Read the model definition and answer for the solid it produces. Units are mm, in the model's axes. Coordinates: 2 decimals unless noted, no trailing zeros. Write each loop counter-clockwise with the first axis right and the second up, starting at its lowest first coordinate (ties: lowest second). Pieces come first, ordered by that corner, then holes.
(1) The mould has two halves that part along X. Classify faces 1 (the flat face through (0, 2, 1)), 2 (the cylindrical face through (0.148, 0.986, 5.752)), 3 (the cylindrical face through (9.5, 0.99, -0.07)), 4 (the cylindrical face through (0.093, 0.986, -0.247)): +X half, -X half, draft (parallel to the pull), parting line (faces both ways), or undercut.
(2) Given pin 1 (3.5 mm diameter, centred on x = -8, z = 0, fed in from -Y), flat-ended and moving along its own axis, determine where the tip first touches the part or whether it passes through.
(3) Section B-B on x = 7 is taken. Write down the section's boundary in (y, z), then the cut area to 3 significant figures.
(4) Find the intervals of material crossed by probe 1 along X at (y, z) = (1.75, 0.25); probe 2 along X at (y, z) = (1.45, 1.25); probe 3 along Z at (x, y) = (8, 0.5), in increasing order.
(5) Section A-A on z = 0 is taken. Write down the section's boundary in (x, y), then the cut area to 3 significant figures.
(6) Section D-D on x = -8 is taken. Write down the section's boundary in (y, z).
Autodesk Inventor part; units mm, degrees
ref_plane "YZ Plane" through (0, 0, 0) normal (1, 0, 0) x (0, 1, 0)
ref_plane "XZ Plane" through (0, 0, 0) normal (0, 1, 0) x (-1, 0, 0)
ref_plane "XY Plane" through (0, 0, 0) normal (0, 0, 1) x (1, 0, 0)
sketch "Sketch1" plane through (0, 0, 0) normal (0, 1, 0) x (-1, 0, 0)
  circle A0 centre (8, 0) radius 3
  line L0 (8, 0) -> (-8, 0)
  circle A1 centre (-8, 0) radius 3
  arc A2 (6.1538, -2.3647) -> (-6.1538, -2.3647) centre (0, -10.247) ccw
  line L1 (0, -0.247) -> (0, 5.753)
  arc A3 (9.8462, 2.3647) -> (-9.8462, 2.3647) centre (0, -10.247) ccw
  circle A4 centre (8, 0) radius 1.5
  circle A5 centre (-8, 0) radius 1.5
  point P0 (0, 0)
  dimension "d13" = 16
  dimension "d14" = 6
  dimension "d16" = 6
  dimension "d17" = 3
  dimension "d18" = 3
extrude "Extrusion1" add sketch "Sketch1" along normal blind 2
properties part number "tahlo-neco"
Response:
1. face 1: draft
1. face 2: parting line
1. face 3: undercut
1. face 4: undercut
2. pin 1: stops at y = 0
3. outline: (0, -2.83) - (2, -2.83) - (2, -1.12) - (0, -1.12) - close; (0, 1.12) - (2, 1.12) - (2, 4.14) - (0, 4.14) - close
3. area: 9.47 mm2
4. probe 1: x = -10.99 to -9.48, -6.52 to 6.52, 9.48 to 10.99
4. probe 2: x = -10.73 to -8.83, -7.17 to 7.17, 8.83 to 10.73
4. probe 3: z = -3 to -1.5, 1.5 to 3.61
5. outline: (-11, 0) - (-9.5, 0) - (-9.5, 2) - (-11, 2) - close; (-6.5, 0) - (6.5, 0) - (6.5, 2) - (-6.5, 2) - close; (9.5, 0) - (11, 0) - (11, 2) - (9.5, 2) - close
5. area: 32.0 mm2
6. outline: (0, -3) - (2, -3) - (2, -1.5) - (0, -1.5) - close; (0, 1.5) - (2, 1.5) - (2, 3.61) - (0, 3.61) - close
